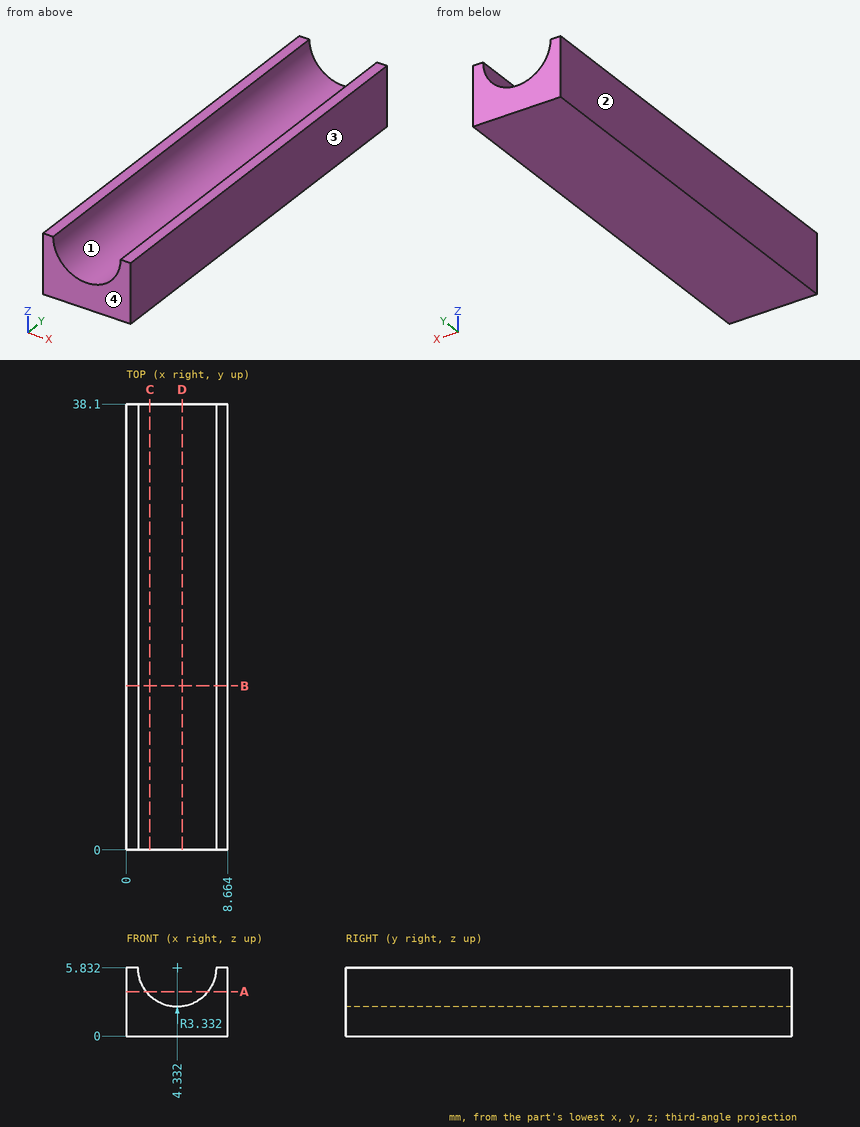
Design review of the part shown in the three views and the two pictorial views. Dimensions are in mm from the part's minimum x, y and z. Give positions to 0.01 mm unless a question says otherwise; leave off trailing zeros. Write each loop counter-clockwise with the first axis right and the second up, starting at its lowest first coordinate (ties: lowest second). Pieces come first, ordered by that corner, then holes. Notation, with made-up numbers: (-18.75, 37) - (19.25, 37) arc R13 cw to (19.25, 51) - close; hole circle Ø6 at (4, 84.25). An arc over 180 degrees is marked (long way). Return JSON: item names as keys, results as strings. Group by question number.
(1) We need section B-B, the plane y = 14. Give the boundary of the cut face in (x, z).
(2) We need section D-D, the plane x = 4.75. Give the boundary of the cut face in (y, z).
(3) Insertion check: pin 1 (1 mm diameter, centred on x = 3, y = 7, fed in from -Z). The pin has a flat end and moves straight along its axis. Give the tip position at first contact, or say it passes through.
(4) We need section A-A, the plane z = 3.8. Give the boundary of the cut face in (x, y).
(5) Mouldability with a two-part tool opening along X and no side actions: class the marked faces 1, 2, 3 and 4 as +X half, -X half, draft (parallel to the pull), parting line (faces both ways), or undercut.
(6) We need section C-C, the plane x = 2. Give the boundary of the cut face in (y, z).
(7) To check wall thickness, follow probe 1 along X at (y, z) = (36.5, 5.3); probe 2 along X at (y, z) = (12.5, 4.45) (1 decimal); probe 3 along Z at (x, y) = (6, 15.5). State the ranges of each line that lie inside material, in increasing order.
Reported:
{
 "1": {"outline": "(0, 0) - (8.66, 0) - (8.66, 5.83) - (7.66, 5.83) arc R3.33 cw to (1, 5.83) - (0, 5.83) - close"},
 "2": {"outline": "(0, 0) - (38.1, 0) - (38.1, 2.53) - (0, 2.53) - close"},
 "3": {"pin 1": "stops at z = 0"},
 "4": {"outline": "(0, 0) - (1.69, 0) - (1.69, 38.1) - (0, 38.1) - close; (6.97, 0) - (8.66, 0) - (8.66, 38.1) - (6.97, 38.1) - close"},
 "5": {"face 1": "undercut", "face 2": "-X half", "face 3": "+X half", "face 4": "draft"},
 "6": {"outline": "(0, 0) - (38.1, 0) - (38.1, 3.45) - (0, 3.45) - close"},
 "7": {"probe 1": "x = 0 to 1.04, 7.62 to 8.66", "probe 2": "x = 0 to 1.3, 7.4 to 8.7", "probe 3": "z = 0 to 2.95"}
}
